from build123d import *

# Parameters (mm, degrees)
F0_R     = 4.15
F1_DEPTH = 41.7
F2_R     = 1.75
F3_DEPTH = 0.8
F4_R     = 0.5
F5_R     = 0.5
F6_R     = 0.3


with BuildPart() as f1:
    # F0 (on Top) → F1 (new body)
    with BuildSketch(Plane.XY):
        Circle(F0_R)
    extrude(amount=F1_DEPTH)

    # F2 (on face) → F3 (join)
    with BuildSketch(Plane(origin=(0, 0, 0), x_dir=(1, 0, 0), z_dir=(0, 0, -1))):
        Circle(F2_R)
    extrude(amount=F3_DEPTH)

    # F4
    f4_edges = [f1.edges().sort_by_distance(p)[0] for p in [
        (-4.15, 0, 0),
    ]]
    fillet(f4_edges, radius=F4_R)

    # F5
    f5_edges = [f1.edges().sort_by_distance(p)[0] for p in [
        (-4.15, 0, 41.7),
    ]]
    fillet(f5_edges, radius=F5_R)

    # F6
    f6_edges = [f1.edges().sort_by_distance(p)[0] for p in [
        (-1.75, 0, -0.8),
        (-1.75, 0, 0),
    ]]
    fillet(f6_edges, radius=F6_R)


solid = f1.part
The model under review builds one solid part; all positions refer to its coordinate system, in mm. A direction names the side the tool comes from. Coordinates: 2 decimals unless noted, no trailing zeros. Loops run counter-clockwise (first coordinate to the right, second up) from the corner with the lowest first, then second, coordinate; pieces in that order, holes last. Notation, with made-up numbers: M -34.75,-17 L 24.25,-17 A17 cw 24.25,4 Z; hole C 44,-37 d10. An arc over 180 degrees is marked long. Put each result on its own line as item: value. Start each with the question number.
Q1. Wall thickness on line 1 (Z direction, x = 3, y = 2); line 2 (X direction, y = 0.25, z = 28.5): over which ranges is each line inside the solid? List them lowest first.
Q2. For faces 1 (the flat face through (0, 0, 41.7)), 2 (the flat face through (2, -2, 0)), list the 3-axis set-ups (+Z, -Z, +X, -X, +Y, -Y) from which the entire face can be reached by the end or side of a thin tool; tool diameter is ignored.
Q3. Add section A-A (z = 22.5). Write out the cut boundary in (x, y).
Q4. Clearance check with flat-ended pins moving along their axes: pin 1 (4 mm diameter, centred on x = 1, z = 21.5, fed in from +Y); pin 2 (4 mm diameter, centred on y = 3, z = 9, fed in from +X); pin 3 (1.5 mm diameter, centred on x = -2, z = 31, fed in from -Y); pin 4 (1.5 mm diameter, centred on x = 2, y = -2.5, fed in from -Z). State where each tip first meets the part, or that it passes through.
Answers:
1. line 1: z = 0 to 41.7
1. line 2: x = -4.14 to 4.14
2. face 1: +Z, +X, -X, +Y, -Y
2. face 2: -Z
3. outline: C 0,0 d8.3
4. pin 1: stops at y = 4.15
4. pin 2: stops at x = 4.03
4. pin 3: stops at y = -3.96
4. pin 4: stops at z = 0
